Geometry check sheet. Reference: the model listing, model coordinates, mm. Coordinates: 2 decimals unless noted, no trailing zeros. Order: outer loops, then holes, each group sorted by start corner. A loop starts at its lowest first (then second) coordinate and runs counter-clockwise, first axis right, second up.
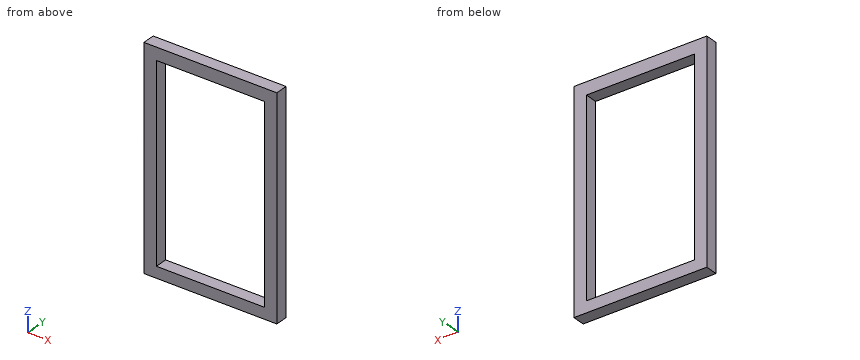
```python
from build123d import *

# Parameters (mm, degrees)
F0_W     = 38.1
F0_H     = 38.1
F1_DEPTH = 660.4
F2_W     = 38.1
F2_H     = 38.1
F3_DEPTH = 330.2
F4_W     = 38.1
F4_H     = 34.3169383705
F5_DEPTH = 330.2
F6_W     = 38.1
F6_H     = 38.1
F7_DEPTH = 660.4


with BuildPart() as f1:
    # F0 (on Top) → F1 (new body)
    with BuildSketch(Plane.XY):
        Rectangle(F0_W, F0_H)
    extrude(amount=F1_DEPTH)

    # F2 (on face) → F3 (join)
    with BuildSketch(Plane.YZ.offset(19.05)):
        with Locations((0, 641.35)):
            Rectangle(F2_W, F2_H)
    extrude(amount=F3_DEPTH)

    # F4 (on face) → F5 (join)
    with BuildSketch(Plane.YZ.offset(19.05)):
        with Locations((0, 17.1584691852)):
            Rectangle(F4_W, F4_H)
    extrude(amount=F5_DEPTH)

    # F6 (on face) → F7 (join)
    with BuildSketch(Plane(origin=(0, 0, 0), x_dir=(1, 0, 0), z_dir=(0, 0, -1))):
        with Locations((368.3, 0)):
            Rectangle(F6_W, F6_H)
    extrude(amount=-F7_DEPTH)


solid = f1.part
```
Item 1: Sectioned sample at B-B (x = 92). Record the cut outline in (y, z), and give its area (3 significant figures).
Item 2: Thickness scan on line 1 along Z through (x, y) = (172, 6.5); line 2 along X through (y, z) = (0.5, 322). Record the ranges inside material, lowest first.
Item 3: Sectioned sample at A-A (z = 68.5). Record the cut outline in (x, y), and give its area (3 significant figures).
Item 4: Sectioned sample at C-C (y = 9). Record the cut outline in (x, z), and give its area (3 significant figures).
Geometry check:
1. outline: (-19.05, 0) - (19.05, 0) - (19.05, 34.32) - (-19.05, 34.32) - close; (-19.05, 622.3) - (19.05, 622.3) - (19.05, 660.4) - (-19.05, 660.4) - close
1. area: 2,760 mm2
2. line 1: z = 0 to 34.32, 622.3 to 660.4
2. line 2: x = -19.05 to 19.05, 349.25 to 387.35
3. outline: (-19.05, -19.05) - (19.05, -19.05) - (19.05, 19.05) - (-19.05, 19.05) - close; (349.25, -19.05) - (387.35, -19.05) - (387.35, 19.05) - (349.25, 19.05) - close
3. area: 2,900 mm2
4. outline: (-19.05, 0) - (387.35, 0) - (387.35, 660.4) - (-19.05, 660.4) - close; hole (19.05, 34.32) - (349.25, 34.32) - (349.25, 622.3) - (19.05, 622.3) - close
4. area: 74,200 mm2
